Autodesk Fusion 360 part; units mm, degrees
sketch "Sketch1" plane through (0, 0, 0) normal (0, 0, 1) x (1, 0, 0)
  line L0 (0, 0) -> (195, 0)
  line L1 (195, 0) -> (195, 140)
  line L2 (195, 140) -> (0, 140)
  line L3 (0, 140) -> (0, 0)
  line L4 (60, 140) -> (60, 0)
  line L5 (135, 140) -> (135, 0)
  circle A0 centre (68.5, 10) radius 1.7
  circle A1 centre (126.5, 10) radius 1.7
  line L6 (97.5, 0) -> (97.5, 140) construction
  circle A2 centre (68.5, 130) radius 1.7
  circle A3 centre (126.5, 130) radius 1.7
  line L7 (68.5, 130) -> (68.5, 100) construction
  circle A4 centre (68.5, 107) radius 1.7
  line L8 (126.5, 130) -> (126.5, 100) construction
  circle A5 centre (126.5, 107) radius 1.7
  circle A6 centre (48, 120) radius 2
  line L9 (0, 70) -> (195, 70) construction
  circle A7 centre (48, 20) radius 2
  circle A8 centre (147, 120) radius 2
  circle A9 centre (147, 20) radius 2
  line L10 (50, 0) -> (50, 140) construction
  line L11 (145, 0) -> (145, 140) construction
  circle A10 centre (55, 10) radius 1.7
  circle A11 centre (55, 130) radius 1.7
  circle A12 centre (140, 130) radius 1.7
  circle A13 centre (140, 10) radius 1.7
  dimension "d1" = 140
  dimension "d3" = 60
  dimension "d4" = 60
  dimension "d5" = 3.4
  dimension "d6" = 10
  dimension "d7" = 3.4
  dimension "d10" = 58
  dimension "d11" = 3.4
  dimension "d12" = 3.4
  dimension "d13" = 58
  dimension "d14" = 10
  dimension "d23" = 3.4
  dimension "d24" = 23
  dimension "d25" = 3.4
  dimension "d26" = 23
  dimension "d27" = 4
  dimension "d28" = 4
  dimension "d29" = 100
  dimension "d30" = 4
  dimension "d31" = 4
  dimension "d32" = 100
  dimension "d42" = 75
  dimension "d43" = 50
  dimension "d44" = 50
  dimension "d46" = 3.4
  dimension "d47" = 10
  dimension "d48" = 3.4
  dimension "d49" = 10
  dimension "d50" = 3.4
  dimension "d51" = 10
  dimension "d52" = 3.4
  dimension "d53" = 10
  dimension "d54" = 5
  dimension "d55" = 5
  dimension "d56" = 5
  dimension "d57" = 5
extrude "Extrude1" add sketch "Sketch1" along normal blind 20 contours L0 L2 L4 L5
extrude "Extrude3" add sketch "Sketch1" along normal blind 5 contours L0 L2 L3 L4 | L0 L1 L2 L5
extrude "Extrude4" add sketch "Sketch1" along normal blind 15 contours A0 | A1
extrude "Extrude5" add sketch "Sketch1" along normal blind 10 from surface at 5 contours A2 | A3
extrude "Extrude6" add sketch "Sketch1" along normal blind 15 from surface at 5 contours A4 | A5
equation "d5 = m3_hole_diameter"
equation "d7 = m3_hole_diameter"
equation "d11 = m3_hole_diameter"
equation "d12 = m3_hole_diameter"
equation "d23 = m3_hole_diameter"
equation "d25 = m3_hole_diameter"
equation "d27 = zip_tie_hole_diameter"
equation "d28 = zip_tie_hole_diameter"
equation "d30 = zip_tie_hole_diameter"
equation "d31 = zip_tie_hole_diameter"
equation "zip_tie_hole_diameter = 4 mm"
equation "m3_hole_diameter = 3.4 mm"
equation "d46 = m3_hole_diameter"
equation "d48 = m3_hole_diameter"
equation "d50 = m3_hole_diameter"
equation "d52 = m3_hole_diameter"
Work out the finished part from the listing and answer in its coordinate system (mm). A direction names the side the tool comes from. Coordinates: 2 decimals unless noted, no trailing zeros. Write each loop counter-clockwise with the first axis right and the second up, starting at its lowest first coordinate (ties: lowest second). Pieces come first, ordered by that corner, then holes.
Q1. A cutting plane is placed at D-D, the plane z = 11.5. Give the vertices of the cut face in (x, y).
Q2. Which of the six approach directions +Z, -Z, +X, -X, +Y, -Y give full straight-line access (tool end or side, diameter ignored) to faces 4 (the face through (165, 71, 5)), 5 (the face through (195, 69, 2)), 6 (the face through (30, 71, 5))?
Q3. A cutting plane is placed at A-A, the plane x = 147. Give the vertices of the cut face in (y, z), then the cut area to 3 significant figures.
Q4. Determine the mould class of faces 1 (the face through (96, 0, 8)), 2 (the face through (49.075, 118.314, 2.465)), 3 (the face through (135, 71, 12)) for opening direction X: released by +X, released by -X, zero draft, split by the parting line, or undercut.
Q5. Find the intervals of material crossed by line 1 (X direction, y = 107, z = 1.7); line 2 (Y direction, x = 48, z = 1.9); line 3 (X direction, y = 130, z = 3.3), in increasing order.
Q6. A cutting plane is placed at B-B, the plane y = 20. Give the vertices of the cut face in (x, z), then the cut area to 3 significant figures.
Q7. Each of these flat-tipped pins is pushed along its axis until it touches: pin 1 Ø1.5 at (y, z) = (83, 14) entering from -X; pin 2 Ø2.5 at (x, y) = (68.5, 130) entering from -Z; pin 3 Ø5 at (x, y) = (48, 20) entering from +Z. Where does it stop, or does it pass through?
Q8. A cutting plane is placed at C-C, the plane x = 34. Give the vertices of the cut face in (y, z), then the cut area to 3 significant figures.
Findings below:
1. outline: (60, 0) - (135, 0) - (135, 140) - (60, 140) - close
2. face 4: +Z, +X, +Y, -Y
2. face 5: +Z, -Z, +X, +Y, -Y
2. face 6: +Z, -X, +Y, -Y
3. outline: (0, 0) - (18, 0) - (18, 5) - (0, 5) - close; (22, 0) - (118, 0) - (118, 5) - (22, 5) - close; (122, 0) - (140, 0) - (140, 5) - (122, 5) - close
3. area: 660 mm2
4. face 1: zero draft
4. face 2: undercut
4. face 3: released by +X
5. line 1: x = 0 to 66.8, 70.2 to 124.8, 128.2 to 195
5. line 2: y = 0 to 18, 22 to 118, 122 to 140
5. line 3: x = 0 to 53.3, 56.7 to 66.8, 70.2 to 124.8, 128.2 to 138.3, 141.7 to 195
6. outline: (0, 0) - (46, 0) - (46, 5) - (0, 5) - close; (50, 0) - (145, 0) - (145, 5) - (135, 5) - (135, 20) - (60, 20) - (60, 5) - (50, 5) - close; (149, 0) - (195, 0) - (195, 5) - (149, 5) - close
6. area: 2,060 mm2
7. pin 1: stops at x = 60
7. pin 2: stops at z = 5
7. pin 3: stops at z = 5
8. outline: (0, 0) - (140, 0) - (140, 5) - (0, 5) - close
8. area: 700 mm2
